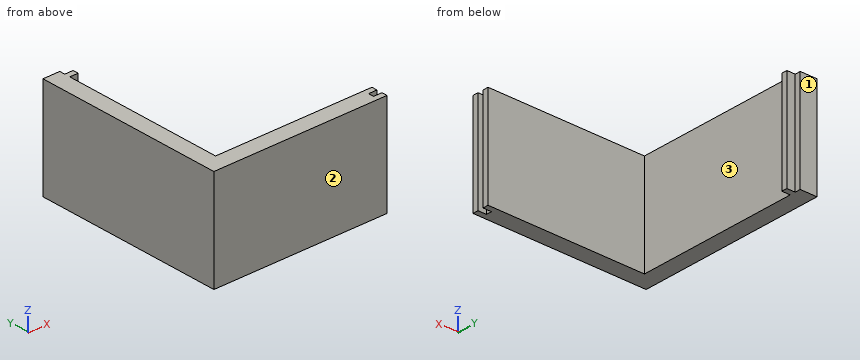
```python
from build123d import *

# Parameters (mm, degrees)
BOSS_EXTRUDE_EQUERRE_DEPTH = 18
ESQUISSE2_W                = 3
ESQUISSE2_H                = 1
ENL_V_MAT_EXTRU_1_DEPTH    = 19
ESQUISSE3_W                = 1.5
ESQUISSE3_H                = 1
BOSS_EXTRU_1_DEPTH         = 18


with BuildPart() as part:
    # Esquisse1 → Boss_Extrude_Equerre (new body)
    with BuildSketch(Plane(origin=(0, 0, 0), x_dir=(0, 1, 0), z_dir=(0, 0, 1))):
        Polygon((0, 0), (31, 0), (31, 3), (-3, 3), (-3, 0), (-3, -28), (0, -28), align=None)
    extrude(amount=BOSS_EXTRUDE_EQUERRE_DEPTH)

    # Esquisse2 → Enlèv. mat.-Extru.1 (cut, through all)
    with BuildSketch(Plane.XY.offset(18)):
        with Locations((28, -1.5)):
            Rectangle(ESQUISSE2_W, ESQUISSE2_H)
    extrude(amount=-ENL_V_MAT_EXTRU_1_DEPTH, mode=Mode.SUBTRACT)

    # Esquisse3 → Boss.-Extru.1 (add, through all)
    with BuildSketch(Plane.XY.offset(18)):
        with Locations((0.75, 29.5)):
            Rectangle(ESQUISSE3_W, ESQUISSE3_H)
    extrude(amount=-BOSS_EXTRU_1_DEPTH)


solid = part.part
```
Could you check a few things on this model? Use its own coordinates, in mm. Face numbers are marked on the shaded views. Coordinates: 2 decimals unless noted, no trailing zeros. Loops run counter-clockwise (first coordinate to the right, second up) from the corner with the lowest first, then second, coordinate; pieces in that order, holes last.
1) Imagine slicing it at A-A (z = 11). List the corners of the cut face in (x, y) for me.
Reported:
outline: (-3, -3) - (28, -3) - (28, -2) - (26.5, -2) - (26.5, -1) - (28, -1) - (28, 0) - (0, 0) - (0, 29) - (1.5, 29) - (1.5, 30) - (0, 30) - (0, 31) - (-3, 31) - close
2) Thinking about a two-plate mould opening in Y: for the marked faces 1, 2 and 3, which applies, released by +Y, released by -Y, zero draft, split by the parting line, or undercut?
Reported:
face 1: released by +Y
face 2: released by -Y
face 3: undercut
3) Please list where these lines run through material, in increasing order: line 1 along Y through (x, z) = (27.5, 9.25); line 2 along X through (y, z) = (23, 13.25).
Reported:
line 1: y = -3 to -2, -1 to 0
line 2: x = -3 to 0
4) Imagine slicing it at B-B (x = 16.5). List the corners of the cut face in (y, z) for me.
Reported:
outline: (-3, 0) - (0, 0) - (0, 18) - (-3, 18) - close
5) Will these pins go through, and if not, where does the flat tip stop? pin 1 Ø0.8 at (x, z) = (27, 10.5) entering from +Y; pin 2 Ø0.8 at (y, z) = (30.5, 10) entering from +X; pin 3 Ø0.8 at (y, z) = (29.5, 8) entering from +X.
Reported:
pin 1: stops at y = 0
pin 2: stops at x = 0
pin 3: stops at x = 1.5
